```python
from build123d import *

# Parameters (mm, degrees)
BOSS_EXTRUDE1_DEPTH     = 6.35
SKETCH2_R               = 2
CUT_EXTRUDE1_DEPTH      = 1
CUT_EXTRUDE1_DEPTH_BACK = 83.55
FILLET1_R               = 2.54
M4_CLEARANCE_HOLE1_D    = 4.3


with BuildPart() as part:
    # Sketch1 → Boss-Extrude1 (new body)
    with BuildSketch(Plane(origin=(0, 0, 0), x_dir=(1, 0, 0), z_dir=(0, 1, 0))):
        Polygon((0, 0), (63.5, 0), (63.5, 6.35), (50.8, 6.35), (50.8, 82.55), (12.7, 82.55), (12.7, 6.35), (0, 6.35), align=None)
    extrude(amount=BOSS_EXTRUDE1_DEPTH)

    # Sketch2 → Cut-Extrude1 (cut, two sides)
    with BuildSketch(Plane.XY) as cut_extrude1_sk:
        with Locations((6.35, 3.175)):
            Circle(SKETCH2_R)
        with Locations((57.15, 3.175)):
            Circle(SKETCH2_R)
    extrude(amount=CUT_EXTRUDE1_DEPTH, mode=Mode.SUBTRACT)
    extrude(cut_extrude1_sk.sketch, amount=-CUT_EXTRUDE1_DEPTH_BACK, mode=Mode.SUBTRACT)

    # Fillet1
    fillet1_edges = [part.edges().sort_by_distance(p)[0] for p in [
        (12.7, 3.175, -6.35),
        (50.8, 3.175, -6.35),
    ]]
    fillet(fillet1_edges, radius=FILLET1_R)

    # M4 Clearance Hole1 (through all)
    with Locations(Plane(origin=(0, 6.35, 0), x_dir=(1, 0, 0), z_dir=(0, 1, 0))):
        with Locations((17.4625, 77.7875), (46.0375, 77.7875), (46.0375, 26.9875), (17.4625, 26.9875)):
            Hole(M4_CLEARANCE_HOLE1_D / 2)


solid = part.part
```
Design review of the part built by this model. Coordinates are the model's own, in mm. A direction names the side the tool comes from. Give positions to 0.01 mm unless a question says otherwise; leave off trailing zeros. Write each loop counter-clockwise with the first axis right and the second up, starting at its lowest first coordinate (ties: lowest second). Pieces come first, ordered by that corner, then holes.
(1) Wall thickness on line 1 along X through (y, z) = (3.75, -26); line 2 along X through (y, z) = (1.5, -35.5); line 3 along Z through (x, y) = (7, 5.75): over which ranges is each line inside the solid? List them lowest first.
Checked values:
line 1: x = 12.7 to 15.55, 19.37 to 44.13, 47.95 to 50.8
line 2: x = 12.7 to 50.8
line 3: z = -6.35 to 0
(2) Mouldability with a two-part tool opening along X and no side actions: class faces 4 (the face through (63.5, 3, -3)), 5 (the face through (55.68, 4.53, -3.13)), 6 (the face through (31, 3, 0)), 7 (the face through (43.987, 3.131, -27.633)) as +X half, -X half, draft (parallel to the pull), parting line (faces both ways), or undercut.
Checked values:
face 4: +X half
face 5: undercut
face 6: draft
face 7: undercut
(3) Add section B-B (x = 18). Give the boundary of the cut face in (y, z), and give its area (3 significant figures).
Checked values:
outline: (0, -82.55) - (6.35, -82.55) - (6.35, -79.87) - (0, -79.87) - close; (0, -75.71) - (6.35, -75.71) - (6.35, -29.07) - (0, -29.07) - close; (0, -24.91) - (6.35, -24.91) - (6.35, 0) - (0, 0) - close
area: 471 mm2
(4) Add section A-A (x = 57.15). Give the boundary of the cut face in (y, z) (3 decimals).
Checked values:
outline: (0, -6.35) - (1.175, -6.35) - (1.175, 0) - (0, 0) - close; (5.175, -6.35) - (6.35, -6.35) - (6.35, 0) - (5.175, 0) - close
(5) Add section C-C (z = -51.5). Give the boundary of the cut face in (x, y), and give its area (3 significant figures).
Checked values:
outline: (12.7, 0) - (50.8, 0) - (50.8, 6.35) - (12.7, 6.35) - close
area: 242 mm2
(6) Tool access review of faces 1 (the face through (60, 3, -6.35)), 2 (the face through (32, 3, -82.55)), 3 (the face through (4, 3, -6.35)): name each direction out of +Z, -Z, +X, -X, +Y, -Y from which nothing blocks a thin tool from reaching the whole face with its end or side.
Checked values:
face 1: -Z, +X, +Y, -Y
face 2: -Z, +X, -X, +Y, -Y
face 3: -Z, -X, +Y, -Y
(7) Clearance check with flat-ended pins moving along their axes: pin 1 Ø4 at (x, z) = (46.04, -26.99) entering from +Y; pin 2 Ø1.9 at (x, y) = (4.5, 4) entering from -Z; pin 3 Ø3 at (y, z) = (4, -59) entering from -X. State where each tip first meets the part, or that it passes through.
Checked values:
pin 1: passes through
pin 2: stops at z = -6.35
pin 3: stops at x = 12.7
